Source: CAD feature listing. Evaluate the final solid. Frame: model axes, mm. A direction names the side the tool comes from. Round coordinates to 2 decimals unless told otherwise and drop trailing zeros. Order: outer loops, then holes, each group sorted by start corner. A loop starts at its lowest first (then second) coordinate and runs counter-clockwise, first axis right, second up. Notation, with made-up numbers: M -6.5,8.25 L 35.5,8.25 A11 cw 35.5,20.25 Z; hole C 89.25,33.25 d2. An arc over 180 degrees is marked long. Use CSV: the item, a comma, the result in double quotes. Start each with the question number.
```python
from build123d import *

# Parameters (mm, degrees)
SKETCH2_W           = 100
SKETCH2_H           = 100
BOSS_EXTRUDE1_DEPTH = 75
SHELL1_T            = -10
SKETCH3_W           = 90
SKETCH3_H           = 90
CUT_EXTRUDE1_DEPTH  = 5


with BuildPart() as part:
    # Sketch2 → Boss-Extrude1 (new body)
    with BuildSketch(Plane.XY):
        Rectangle(SKETCH2_W, SKETCH2_H)
    extrude(amount=BOSS_EXTRUDE1_DEPTH)

    # Shell1
    shell1_openings = [part.faces().sort_by_distance(p)[0] for p in [
        (0, 0, 75),
    ]]
    offset(amount=SHELL1_T, openings=shell1_openings, kind=Kind.INTERSECTION)

    # Sketch3 → Cut-Extrude1 (cut)
    with BuildSketch(Plane.XY.offset(75)):
        Rectangle(SKETCH3_W, SKETCH3_H)
    extrude(amount=-CUT_EXTRUDE1_DEPTH, mode=Mode.SUBTRACT)


solid = part.part
```
(1) Section A-A on z = 20.5. Return loops of the section in (x, y).
(2) Line query: line 1 along X through (y, z) = (14, 21); line 2 along Z through (x, y) = (11, 5). Output: solid intervals per line, ascending.
(3) Section C-C on x = 41.5. Return loops of the section in (y, z).
(4) Contact query for a flat-ended pin moving along its axis: P1, Ø24, axis at x = 15, y = -0.5, coming from the +Z side. Output: stop coordinate, or through.
(5) Section B-B on y = -14. Return loops of the section in (x, z), plus the area to 3 significant figures.
(6) Draft query along Y for faces 1 (the face through (-1, 45, 73)), 2 (the face through (-4, -48, 75)), 3 (the face through (-1, -50, 37)). Return one class per face: pulls with the +Y half, pulls with the -Y half, needs draft (parallel to the pull), parting line crosses it, or undercut.
(7) Reachability of faces 4 (the face through (-1, -45, 73)), 5 (the face through (-1, 50, 37)) from +Z, -Z, +X, -X, +Y, -Y: full face, straight path, thin tool, end or side. Return the list, or none.
Results below:
1,outline,"M -50,-50 L 50,-50 L 50,50 L -50,50 Z; hole M -40,-40 L 40,-40 L 40,40 L -40,40 Z"
2,line 1,"x = -50 to -40, 40 to 50"
2,line 2,"z = 0 to 10"
3,outline,"M -50,0 L 50,0 L 50,75 L 45,75 L 45,70 L -45,70 L -45,75 L -50,75 Z"
4,P1,"stops at z = 10"
5,outline,"M -50,0 L 50,0 L 50,75 L 45,75 L 45,70 L 40,70 L 40,10 L -40,10 L -40,70 L -45,70 L -45,75 L -50,75 Z"
5,area,"2,250 mm2"
6,face 1,"undercut"
6,face 2,"needs draft"
6,face 3,"pulls with the -Y half"
7,face 4,"+Z"
7,face 5,"+Z, -Z, +X, -X, +Y"
